Autodesk Inventor part; units mm, degrees
ref_plane "YZ Plane" through (0, 0, 0) normal (1, 0, 0) x (0, 1, 0)
ref_plane "XZ Plane" through (0, 0, 0) normal (0, 1, 0) x (-1, 0, 0)
ref_plane "XY Plane" through (0, 0, 0) normal (0, 0, 1) x (1, 0, 0)
sketch "Sketch1" plane through (0, 0, 0) normal (0, 0, 1) x (1, 0, 0)
  circle A0 centre (-14, 4) radius 1.5
  circle A1 centre (-10, 13) radius 1.5
  circle A2 centre (-7, 4) radius 1.5
  line L0 (-20, 0) -> (-20, 8)
  line L1 (0, 0) -> (-20, 0)
  line L2 (0, 40) -> (0, 0)
  line L3 (-10, 40) -> (0, 40)
  line L4 (-10, 23) -> (-10, 40)
  line L5 (-10, 23) -> (-20, 8)
  circle A3 centre (14, 4) radius 1.5
  circle A4 centre (10, 13) radius 1.5
  circle A5 centre (7, 4) radius 1.5
  line L6 (20, 0) -> (20, 8)
  line L7 (10, 23) -> (20, 8)
  line L8 (10, 23) -> (10, 40)
  line L9 (10, 40) -> (0, 40)
  line L10 (0, 40) -> (0, 0)
  line L11 (0, 0) -> (20, 0)
  arc A6 (-12.05, 74.2834) -> (-20, 79.501) centre (-23.25, 65.8834) ccw
  line L12 (-8.0217, 68.9123) -> (-12.05, 74.2834)
  line L13 (-10, 40) -> (-8.0217, 68.9123)
  line L14 (-10, 23) -> (-10, 40)
  line L15 (-20, 8) -> (-10, 23)
  line L16 (-20, -45) -> (-20, 8)
  line L17 (20, -45) -> (-20, -45)
  line L18 (20, 8) -> (20, -45)
  line L19 (10, 23) -> (20, 8)
  line L20 (10, 40) -> (10, 23)
  line L21 (8.0217, 68.9123) -> (10, 40)
  line L22 (12.05, 74.2834) -> (8.0217, 68.9123)
  arc A7 (20, 79.501) -> (12.05, 74.2834) centre (23.25, 65.8834) ccw
  line L23 (20, 86.8834) -> (20, 79.501)
  line L24 (-20, 86.8834) -> (20, 86.8834)
  line L25 (-20, 79.501) -> (-20, 86.8834)
  circle A8 centre (10, 13) radius 1.5
  circle A9 centre (7, 4) radius 1.5
  circle A10 centre (14, 4) radius 1.5
  circle A11 centre (-14, 4) radius 1.5
  circle A12 centre (-7, 4) radius 1.5
  circle A13 centre (-10, 13) radius 1.5
  circle A14 centre (9, 80.8834) radius 1.5
  circle A15 centre (-9, 80.8834) radius 1.5
  line L26 (3, 264.8834) -> (-3, 264.8834)
  line L27 (-3, 264.8834) -> (-3, -35.1166)
  line L28 (3, -35.1166) -> (-3, -35.1166)
  line L29 (3, 264.8834) -> (3, -35.1166)
  line L30 (8.0217, 68.9123) -> (-8.0217, 68.9123)
  line L31 (3, 40) -> (-3, 40)
  line L32 (-3, 40) -> (-3, 68.9123)
  line L33 (-3, 68.9123) -> (3, 68.9123)
  line L34 (3, 68.9123) -> (3, 40)
  circle A16 centre (-7.7386, -39.5) radius 1.5
  circle A17 centre (-15.7386, -39.5) radius 1.5
  circle A18 centre (7.7386, -39.5) radius 1.5
  circle A19 centre (15.7386, -39.5) radius 1.5
  point P0 (-3, 40)
  point P1 (3, 68.9123)
extrude "Extrusion1" add sketch "Sketch1" along normal blind 2 contours L0 L5 L4 L3 L27 L1 | L1 L27 L28 L29 L11 L18 L17 L16 | L27 L3 L2 L1 | L1 L11 L29 L28 L27 | L2 L9 L29 L11 | L27 L30 L29 L9 L3 | L29 L9 L8 L7 L6 L11 | L30 L12 A6 L25 L24 L27 | L27 L24 L29 L30 | L29 L24 L23 A7 L22 L30 | A16 | A17 | A18 | A19
fillet "Fillet1" radius 3 4 edges at (3, 40, 1) (-3, 40, 1) (-3, 68.9123, 1) (3, 68.9123, 1)
sketch "Sketch2" plane through (0, 0, 2) normal (0, 0, 1) x (1, 0, 0)
  circle A0 centre (-7.7386, -39.5) radius 1.5
  circle A1 centre (-15.7386, -39.5) radius 1.5
  point P0 (0, 0)
extrude "Extrusion2" cut sketch "Sketch2" against normal blind 10
ref_plane "Work Plane1" through (0, -45, 0) normal (-1, 0, 0) x (0, 0, 1)
mirror "Mirror1" about plane through (0, -45, 0) normal (-1, 0, 0) of "Extrusion2"
sketch "Sketch3" plane through (0, 0, 2) normal (0, 0, 1) x (1, 0, 0)
  circle A0 centre (15.7386, -39.5) radius 1.5
  circle A1 centre (7.7386, -39.5) radius 1.5
  circle A2 centre (-15.7386, -39.5) radius 1.5
  circle A3 centre (-7.7386, -39.5) radius 1.5
  line L0 (-8.0217, 68.9123) -> (-6, 68.9123)
  arc A4 (-3, 65.9123) -> (-6, 68.9123) centre (-6, 65.9123) ccw
  line L1 (-3, 65.9123) -> (-3, 43)
  arc A5 (-6, 40) -> (-3, 43) centre (-6, 43) ccw
  line L2 (-6, 40) -> (-10, 40)
  line L3 (-10, 40) -> (-10, 23)
  line L4 (-10, 23) -> (-20, 8)
  line L5 (-20, 8) -> (-20, -45)
  line L6 (-20, -45) -> (20, -45)
  line L7 (20, -45) -> (20, 8)
  line L8 (20, 8) -> (10, 23)
  line L9 (10, 23) -> (10, 40)
  line L10 (10, 40) -> (6, 40)
  arc A6 (3, 43) -> (6, 40) centre (6, 43) ccw
  line L11 (3, 43) -> (3, 65.9123)
  arc A7 (6, 68.9123) -> (3, 65.9123) centre (6, 65.9123) ccw
  line L12 (6, 68.9123) -> (8.0217, 68.9123)
  line L13 (8.0217, 68.9123) -> (12.05, 74.2834)
  arc A8 (20, 79.501) -> (12.05, 74.2834) centre (23.25, 65.8834) ccw
  line L14 (20, 79.501) -> (20, 86.8834)
  line L15 (20, 86.8834) -> (-20, 86.8834)
  line L16 (-20, 86.8834) -> (-20, 79.501)
  arc A9 (-12.05, 74.2834) -> (-20, 79.501) centre (-23.25, 65.8834) ccw
  line L17 (-12.05, 74.2834) -> (-8.0217, 68.9123)
  circle A10 centre (-9, 80.8834) radius 1.5
  circle A11 centre (9, 80.8834) radius 1.5
  circle A12 centre (-14, 4) radius 1.5
  circle A13 centre (-10, 13) radius 1.5
  circle A14 centre (-7, 4) radius 1.5
  circle A15 centre (7, 4) radius 1.5
  circle A16 centre (10, 13) radius 1.5
  circle A17 centre (14, 4) radius 1.5
  line L18 (-14, 4) -> (-14, -6)
  line L19 (-14, -6) -> (-14, -16)
  line L20 (-14, -16) -> (-14, -31)
  circle A18 centre (-14, -6) radius 1.5
  circle A19 centre (-14, -16) radius 1.5
  circle A20 centre (-14, -31) radius 1.5
  circle A21 centre (-6, -6) radius 1.5
  circle A22 centre (-6, -16) radius 1.5
  circle A23 centre (-6, -31) radius 1.5
  point P0 (0, 0)
  dimension "d7" = 10
  dimension "d8" = 10
  dimension "d9" = 15
  dimension "d10" = 3
  dimension "d11" = 3
  dimension "d12" = 3
  dimension "d15" = 8
extrude "Extrusion3" cut sketch "Sketch3" against normal blind 10 contours A20 | A19 L20 L19 | L19 L20 A19 | A18 L19 L18 | L18 L19 A18 | A21 | A22 | A23
mirror "Mirror2" about plane through (0, -45, 0) normal (-1, 0, 0) of "Extrusion3"
properties part number "body_bone_5"
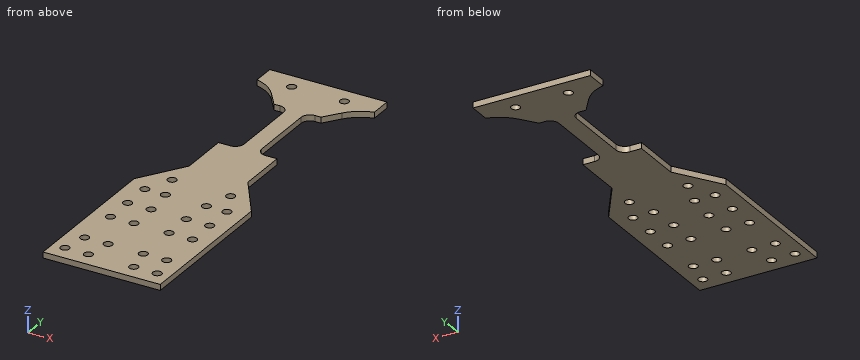
Check sheet for the modelled part. Datum: model origin and axes. Units: mm. Give positions to 0.01 mm unless a question says otherwise; leave off trailing zeros. Loops run counter-clockwise (first coordinate to the right, second up) from the corner with the lowest first, then second, coordinate; pieces in that order, holes last. Notation, with made-up numbers: M 10.25,67 L 29.25,67 A20 ccw 29.25,72 Z; hole C 67,-3.75 d3. An arc over 180 degrees is marked long. Answer as a JSON object with one key per item and string values. Group by question number.
Q1. Cross-section at C-C on y = 55. Record the cut outline in (x, z).
Q2. Cross-section at A-A on y = 4. Record the cut outline in (x, z), then the cut area to 3 significant figures.
Q3. Go/stop test with a flat-tipped pin: P1, Ø1.8, axis at x = -6, y = -6, coming from the -Z side. Record where the tip stops, or that it passes through.
Q4. Cross-section at B-B on z = 0.5. Give the number of separate pieces and of enclosed holes in the cut face, then the cut area to 3 significant figures.
Q5. Material ranges on line 1 along Y through (x, z) = (-9, 0.4); line 2 along Y through (x, z) = (6, 1.5); line 3 along Y through (x, z) = (14, 1.45), recorded low to high. Write a range as [from, to].
Evaluation:
{
 "1": {"outline": "M -3,0 L 3,0 L 3,2 L -3,2 Z"},
 "2": {"outline": "M -20,0 L -15.5,0 L -15.5,2 L -20,2 Z; M -12.5,0 L -8.5,0 L -8.5,2 L -12.5,2 Z; M -5.5,0 L 5.5,0 L 5.5,2 L -5.5,2 Z; M 8.5,0 L 12.5,0 L 12.5,2 L 8.5,2 Z; M 15.5,0 L 20,0 L 20,2 L 15.5,2 Z", "area": "56.0 mm2"},
 "3": {"P1": "passes through"},
 "4": {"separate pieces": "1", "enclosed holes": "24", "area": "3,480 mm2"},
 "5": {"line 1": "y = [-45, -40.31], [-38.69, 11.88], [14.12, 40], [70.22, 79.38], [82.38, 86.88]", "line 2": "y = [-45, -32.5], [-29.5, -17.5], [-14.5, -7.5], [-4.5, 2.88], [5.12, 40], [68.91, 86.88]", "line 3": "y = [-45, -32.5], [-29.5, -17.5], [-14.5, -7.5], [-4.5, 2.5], [5.5, 17], [76.39, 86.88]"}
}
